Model file for the job. Use its own axes, mm. A direction names the side the tool comes from. Give positions to 0.01 mm unless a question says otherwise; leave off trailing zeros. Loops run counter-clockwise (first coordinate to the right, second up) from the corner with the lowest first, then second, coordinate; pieces in that order, holes last. Notation, with made-up numbers: (46, 27) -> (103, 27) arc R21 cw to (103, 35) -> close; hole circle Ø4 at (36, 64.25). An arc over 180 degrees is marked (long way). Use CSV: the item, a comma, the result in double quotes. Start each with the question number.
(1) Drill centre lines: probe 1 along X at (y, z) = (-2.25, -6.25); probe 2 along X at (y, z) = (-6.5, 0.25); probe 3 along Z at (x, y) = (3.5, 9). Where is each one in solid material? Low to high.
(2) Cut at B-B on z = -1. Write the cut outline in (x, y).
(3) Cut at C-C on x = 20. Write the cut outline in (y, z) (3 decimals), then the cut area to 3 significant figures.
(4) Flat gauge pins, fed straight in: pin 1 (4 mm diameter, centred on x = 26.04, y = -2.54, fed in from +Z); pin 2 (1 mm diameter, centred on y = -7, z = 5, fed in from -X); pin 3 (6 mm diameter, centred on x = 7, z = -5, fed in from -Y). Where does each tip first touch, or does it go through?
(5) Pull direction X, two halves, no side cores. Call faces 1 (the cylindrical face through (24.523, -3.018, 6.129)), 2 (the flat face through (3, 4, 9.5)), 3 (the flat face through (28.58, -3, 6)): pulls with the +X half, pulls with the -X half, needs draft (parallel to the pull), parting line crosses it, or undercut.
(6) Cut at D-D on z = 3. Write the cut outline in (x, y), then the cut area to 3 significant figures.
(7) Cut at A-A on x = -19.69. Write the cut outline in (y, z) (3 decimals).
(8) 3-axis set-ups, long thin cutter, end or side, ignore diameter. For faces 4 (the flat face through (19.05, -3, 0)), 5 (the flat face through (5, -2, -5.08)), 6 (the flat face through (-16, 6, 4.765)): which of +Z, -Z, +X, -X, +Y, -Y reach the whole face in a straight line?
from build123d import *
from OCP.BRepFilletAPI import BRepFilletAPI_MakeChamfer

# Parameters (mm, degrees)
SKETCH1_R               = 4.765
BOSS_EXTRUDE1_DEPTH     = 9.5
CHAMFER4_SIZE           = 7.54
CHAMFER4_SIZE2          = 2.54
CHAMFER5_SIZE           = 2.54
CHAMFER5_SIZE2          = 7.62
CUT_EXTRUDE1_DEPTH      = 32.662585176
CUT_EXTRUDE1_DEPTH_BACK = 32.662585176
SKETCH2_W               = 9.53
SKETCH2_H               = 9.53
CUT_EXTRUDE2_DEPTH      = 32.662585176
CUT_EXTRUDE2_DEPTH_BACK = 32.662585176
CUT_EXTRUDE3_DEPTH      = 32.662585236
CUT_EXTRUDE3_DEPTH_BACK = 32.662585236
SKETCH4_R               = 1.59


with BuildPart() as part:
    # Sketch1 → Boss-Extrude1 (new, symmetric)
    with BuildSketch(Plane.XY):
        with BuildLine():
            Line((0, 9.77), (-22.23, 9.77))
            Line((-22.23, 9.77), (-22.23, 4.77))
            Line((-22.23, 4.77), (-9.711509246, -1.067468107))
            ThreePointArc((-9.711509246, -1.067468107), (-5.877874817, -7.804068659), (1.655323868, -9.628748771))
            Line((1.655323868, -9.628748771), (28.58, -5))
            Line((28.58, -5), (28.58, 0))
            Line((28.58, 0), (9.77, 0))
            ThreePointArc((9.77, 0), (6.908433252, 6.908433252), (0, 9.77))
        make_face()
        Circle(SKETCH1_R, mode=Mode.SUBTRACT)
    extrude(amount=BOSS_EXTRUDE1_DEPTH, both=True)

    # Chamfer4
    chamfer4_edges = [part.edges().sort_by_distance(p)[0] for p in [
        (-22.23, 7.27, -9.5),
        (28.58, -2.5, -9.5),
    ]]
    chamfer4_side = [part.faces().sort_by_distance(p)[0] for p in [
        (-11.115, 9.225622585, -9.5),
    ]]
    chamfer(chamfer4_edges, length=CHAMFER4_SIZE, length2=CHAMFER4_SIZE2, reference=chamfer4_side[0])

    # Chamfer5: one chamfer whose edges measure the first distance from different faces: ONE call of the kernel's chamfer builder (chamfer() names one face for all edges)
    chamfer5_edges_1 = [part.edges().sort_by_distance(p)[0] for p in [
        (-22.23, 7.27, 9.5),
    ]]
    chamfer5_side_1 = [part.faces().sort_by_distance(p)[0] for p in [
        (-22.23, 7.27, 1.27),
    ]]
    chamfer5_edges_2 = [part.edges().sort_by_distance(p)[0] for p in [
        (28.58, -2.5, 9.5),
    ]]
    chamfer5_side_2 = [part.faces().sort_by_distance(p)[0] for p in [
        (28.58, -2.5, 1.27),
    ]]
    chamfer5 = BRepFilletAPI_MakeChamfer(part.part.solid().wrapped)
    for e in chamfer5_edges_1:
        chamfer5.Add(CHAMFER5_SIZE, CHAMFER5_SIZE2, e.wrapped, chamfer5_side_1[0].wrapped)  # the first distance lies on this face
    for e in chamfer5_edges_2:
        chamfer5.Add(CHAMFER5_SIZE, CHAMFER5_SIZE2, e.wrapped, chamfer5_side_2[0].wrapped)  # the first distance lies on this face
    add(Compound.cast(chamfer5.Shape()), mode=Mode.REPLACE)

    # Sketch2 → Cut-Extrude1 (cut, two sides: drawn at the far end of the back side and taken through both)
    with BuildSketch(Plane(origin=(0, 0, 0), x_dir=(1, 0, 0), z_dir=(0, 1, 0)).offset(-CUT_EXTRUDE1_DEPTH_BACK)):
        with Locations((-17.465, 0)):
            Rectangle(SKETCH2_W, SKETCH2_H)
        with Locations((23.815, 0)):
            Rectangle(SKETCH2_W, SKETCH2_H)
    extrude(amount=CUT_EXTRUDE1_DEPTH + CUT_EXTRUDE1_DEPTH_BACK, mode=Mode.SUBTRACT)

    # Sketch3 → Cut-Extrude2 (cut, two sides: drawn at the far end of the back side and taken through both)
    with BuildSketch(Plane(origin=(0, 0, 0), x_dir=(1, 0, 0), z_dir=(0, 1, 0)).offset(-CUT_EXTRUDE2_DEPTH_BACK)):
        with BuildLine():
            Line((-3.81, 5.08), (6.35, 5.08))
            ThreePointArc((6.35, 5.08), (11.43, 0), (6.35, -5.08))
            Line((6.35, -5.08), (-3.81, -5.08))
            ThreePointArc((-3.81, -5.08), (-8.89, 0), (-3.81, 5.08))
        make_face()
    extrude(amount=CUT_EXTRUDE2_DEPTH + CUT_EXTRUDE2_DEPTH_BACK, mode=Mode.SUBTRACT)

    # Sketch4 → Cut-Extrude3 (cut, two sides: drawn at the far end of the back side and taken through both)
    with BuildSketch(Plane.XY.offset(-CUT_EXTRUDE3_DEPTH_BACK)):
        with Locations(Location((-19.69, 7.23, 0), (0, 0, 180))):
            Circle(SKETCH4_R)
        with Locations(Location((26.04, -2.54, 0), (0, 0, 180))):
            Circle(SKETCH4_R)
    extrude(amount=CUT_EXTRUDE3_DEPTH + CUT_EXTRUDE3_DEPTH_BACK, mode=Mode.SUBTRACT)


solid = part.part
Check result:
1,probe 1,"-9.51 to -4.2, 4.2 to 24.48, 27.6 to 28.58"
1,probe 2,"11.42 to 19.05"
1,probe 3,"-9.5 to -5.08, 5.08 to 9.5"
2,outline,"(-12.7, 0.33) -> (-9.71, -1.07) arc R9.77 ccw to (-8.79, -4.26) -> (-8.79, 9.77) -> (-12.7, 9.77) -> close; (11.33, -7.97) -> (19.05, -6.64) -> (19.05, 0) -> (11.33, 0) -> close"
3,outline,"(-6.475, -9.5) -> (0, -9.5) -> (0, -4.765) -> (-6.475, -4.765) -> close; (-6.475, 4.765) -> (0, 4.765) -> (0, 9.5) -> (-6.475, 9.5) -> close"
3,area,"61.3 mm²"
4,pin 1,"z = 8.47"
4,pin 2,"x = -7.29"
4,pin 3,"y = -9.23"
5,face 1,"undercut"
5,face 2,"needs draft"
5,face 3,"pulls with the +X half"
6,outline,"(-12.7, 0.33) -> (-9.71, -1.07) arc R9.77 ccw to (-7.91, -5.74) -> (-7.91, 9.77) -> (-12.7, 9.77) -> close; (10.45, -8.12) -> (19.05, -6.64) -> (19.05, 0) -> (10.45, 0) -> close"
6,area,"119 mm²"
7,outline,"(3.586, -7.816) -> (5.64, -7.816) -> (5.64, -4.765) -> (3.586, -4.765) -> close; (3.586, 4.765) -> (5.64, 4.765) -> (5.64, 7.807) -> (3.586, 7.807) -> close; (8.82, -7.816) -> (9.77, -7.816) -> (9.77, -4.765) -> (8.82, -4.765) -> close; (8.82, 4.765) -> (9.77, 4.765) -> (9.77, 7.807) -> (8.82, 7.807) -> close"
8,face 4,"+X, +Y, -Y"
8,face 5,"+Y, -Y"
8,face 6,"-X, +Y, -Y"
